from build123d import *

# Parameters (mm, degrees)
BOSS_EXTRUDE1_DEPTH = 38.1
BOSS_EXTRUDE2_DEPTH = 3.175
SKETCH2_R           = 4.826
CUT_EXTRUDE1_DEPTH  = 79.921642198
CHAMFER1_SIZE       = 1.5875


with BuildPart() as part:
    # Sketch1 → Boss-Extrude1 (new body)
    with BuildSketch(Plane.XY):
        with BuildLine():
            ThreePointArc((27.5336, 29.6418), (29.024322516, 29.024322516), (29.6418, 27.5336))
            Line((29.6418, 27.5336), (29.6418, -27.5336))
            ThreePointArc((29.6418, -27.5336), (29.024322516, -29.024322516), (27.5336, -29.6418))
            Line((27.5336, -29.6418), (-27.5336, -29.6418))
            ThreePointArc((-27.5336, -29.6418), (-29.024322516, -29.024322516), (-29.6418, -27.5336))
            Line((-29.6418, -27.5336), (-29.6418, 27.5336))
            ThreePointArc((-29.6418, 27.5336), (-29.024322516, 29.024322516), (-27.5336, 29.6418))
            Line((-27.5336, 29.6418), (27.5336, 29.6418))
        make_face()
    extrude(amount=BOSS_EXTRUDE1_DEPTH)

    # Sketch1_3 → Boss-Extrude2 (add)
    with BuildSketch(Plane.XY):
        with BuildLine():
            Line((27.5336, 31.75), (-27.5336, 31.75))
            ThreePointArc((-27.5336, 31.75), (-30.515045032, 30.515045032), (-31.75, 27.5336))
            Line((-31.75, 27.5336), (-31.75, -27.5336))
            ThreePointArc((-31.75, -27.5336), (-30.515045032, -30.515045032), (-27.5336, -31.75))
            Line((-27.5336, -31.75), (27.5336, -31.75))
            ThreePointArc((27.5336, -31.75), (30.515045032, -30.515045032), (31.75, -27.5336))
            Line((31.75, -27.5336), (31.75, 27.5336))
            ThreePointArc((31.75, 27.5336), (30.515045032, 30.515045032), (27.5336, 31.75))
        make_face()
        with BuildLine():
            Line((27.5336, 29.6418), (-27.5336, 29.6418))
            ThreePointArc((-27.5336, 29.6418), (-29.024322516, 29.024322516), (-29.6418, 27.5336))
            Line((-29.6418, 27.5336), (-29.6418, -27.5336))
            ThreePointArc((-29.6418, -27.5336), (-29.024322516, -29.024322516), (-27.5336, -29.6418))
            Line((-27.5336, -29.6418), (27.5336, -29.6418))
            ThreePointArc((27.5336, -29.6418), (29.024322516, -29.024322516), (29.6418, -27.5336))
            Line((29.6418, -27.5336), (29.6418, 27.5336))
            ThreePointArc((29.6418, 27.5336), (29.024322516, 29.024322516), (27.5336, 29.6418))
        make_face(mode=Mode.SUBTRACT)
    extrude(amount=BOSS_EXTRUDE2_DEPTH)

    # Sketch2 → Cut-Extrude1 (cut, through all)
    with BuildSketch(Plane(origin=(29.6418, 0, 0), x_dir=(0, 0, -1), z_dir=(1, 0, 0))):
        with Locations(Location((-25.4, -9.525, 0), (0, 0, 90))):
            Circle(SKETCH2_R)
    extrude(amount=-CUT_EXTRUDE1_DEPTH, mode=Mode.SUBTRACT)

    # Chamfer1
    chamfer1_edges = [part.edges().sort_by_distance(p)[0] for p in [
        (0, 29.6418, 38.1),
        (-29.024322516, 29.024322516, 38.1),
        (-29.6418, 0, 38.1),
        (-29.024322516, -29.024322516, 38.1),
        (0, -29.6418, 38.1),
        (29.024322516, -29.024322516, 38.1),
        (29.6418, 0, 38.1),
        (29.024322516, 29.024322516, 38.1),
    ]]
    chamfer(chamfer1_edges, length=CHAMFER1_SIZE)


solid = part.part
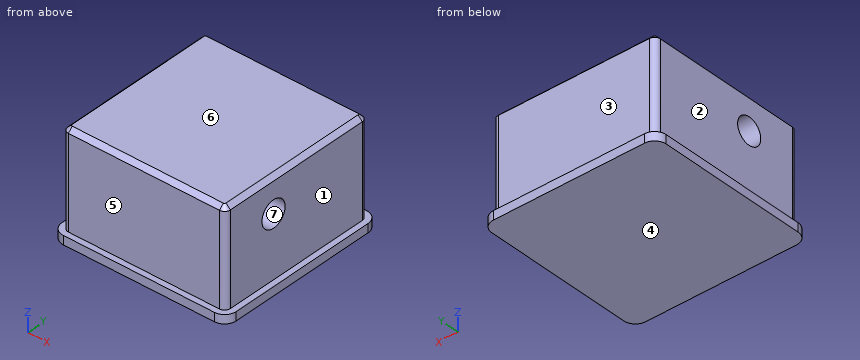
Verification items for the finished model (mm, model axes). Face numbers are marked on the shaded views. A direction names the side the tool comes from. Coordinates: 2 decimals unless noted, no trailing zeros. Order: outer loops, then holes, each group sorted by start corner. A loop starts at its lowest first (then second) coordinate and runs counter-clockwise, first axis right, second up. Notation, with made-up numbers: (21, 9.25) -> (27, 9.25) arc R38 cw to (27, 48.25) -> close; hole circle Ø2 at (-16.5, -0.75). An arc over 180 degrees is marked (long way). Use CSV: the item, a comma, the result in double quotes. Start each with the question number.
Q1. Section check B-B, the plane z = 25.4. Record the cut outline in (x, y), and give its area (3 significant figures).
Q2. Section check D-D, the plane z = 34. Record the cut outline in (x, y).
Q3. Tool access check on the marked faces 1, 2 and 3. Record the directions out of +Z, -Z, +X, -X, +Y, -Y that give a thin tool (end or side, any length) a straight path to the whole face; none if there is none.
Q4. Depth check by flat-ended pin: P1, Ø8, axis at x = -7, z = 8.5, coming from the +Y side; P2, Ø6, axis at y = 19.5, z = 20, coming from the -X side; P3, Ø12, axis at y = 10.5, z = 12.5, coming from the +X side; P4, Ø7.5, axis at y = -9.525, z = 25.4, coming from the -X side (3 decimals). Enter the tip coordinate at first touch or a pass-through.
Q5. Draft check along Z on the marked faces 4, 5, 6 and 7. Enter one of: +Z half, -Z half, draft (parallel to the pull), parting line (faces both ways), or undercut.
Q6. Thickness scan on line 1 along Y through (x, z) = (1, 25); line 2 along X through (y, z) = (19, 21). Record the ranges inside material, lowest first.
Returned:
1,outline,"(-29.64, -27.53) arc R2.11 ccw to (-27.53, -29.64) -> (27.53, -29.64) arc R2.11 ccw to (29.64, -27.53) -> (29.64, -14.35) -> (-29.64, -14.35) -> close; (-29.64, -4.7) -> (29.64, -4.7) -> (29.64, 27.53) arc R2.11 ccw to (27.53, 29.64) -> (-27.53, 29.64) arc R2.11 ccw to (-29.64, 27.53) -> close"
1,area,"2,940 mm^2"
2,outline,"(-29.64, -27.53) arc R2.11 ccw to (-27.53, -29.64) -> (27.53, -29.64) arc R2.11 ccw to (29.64, -27.53) -> (29.64, 27.53) arc R2.11 ccw to (27.53, 29.64) -> (-27.53, 29.64) arc R2.11 ccw to (-29.64, 27.53) -> close"
3,face 1,"+Z, +X, +Y, -Y"
3,face 2,"+Z, -X, +Y, -Y"
3,face 3,"+Z, +X, -X, +Y"
4,P1,"stops at y = 29.64"
4,P2,"stops at x = -29.64"
4,P3,"stops at x = 29.64"
4,P4,"passes through"
5,face 4,"-Z half"
5,face 5,"draft"
5,face 6,"+Z half"
5,face 7,"undercut"
6,line 1,"y = -29.64 to -14.33, -4.72 to 29.64"
6,line 2,"x = -29.64 to 29.64"
